Could you check a few things on this model? Use its own coordinates, in mm. Face numbers are marked on the shaded views. Give positions to 0.01 mm unless a question says otherwise; leave off trailing zeros. Order: outer loops, then holes, each group sorted by start corner. A loop starts at its lowest first (then second) coordinate and runs counter-clockwise, first axis right, second up. Notation, with made-up numbers: (-38.5, -13) - (-12.5, -13) arc R12 cw to (-12.5, 3) - close; hole circle Ø9 at (87, 76.25). An arc over 180 degrees is marked (long way). One line per question, with ' | ' between items. Start each with the question number.
1. Imagine slicing it at A-A (z = 0). Please give me the cut outline in (x, y).
2. Imagine slicing it at D-D (z = 3.25). Please give me the cut outline in (x, y), and give its area (3 significant figures).
3. I need wall thicknesses on probe 1 along Z at (x, y) = (2.4, 0); probe 2 along Y at (x, z) = (1.75, 1.75); probe 3 along Z at (x, y) = (0.45, 3.5). Which ranges of each line are inside material? Lowest first, please. Write a range as from..to.
4. For P1, Ø0.9, axis at y = 0, z = 0, coming from the +X side; P2, Ø1.5, axis at x = 1, z = -2.5, coming from the -Y side, each with a flat end and sliding along its axis, tell me the tip position at first contact or that it passes through.
5. If we mould it in two halves opening along Z, with no side actions, what happens to the marked faces 1, 2, 3 and 4? For each: released by +Z, released by -Z, zero draft, split by the parting line, or undercut.
```python
from build123d import *

# Parameters (mm, degrees)
SKETCH1_R                 = 5
SKETCH1_R_2               = 1.5
BOSS_EXTRUDE1_DEPTH       = 3
SKETCH2_W                 = 0.580440463
SKETCH2_H                 = 2
SKETCH2_W_2               = 2
SKETCH2_H_2               = 0.580440463
BOSS_EXTRUDE2_DEPTH       = 3
CHAMFER3_SIZE             = 0.2
CHAMFER4_SIZE             = 0.2
BOSS_EXTRUDE3_OUTLINE_R   = 1.5
BOSS_EXTRUDE3_OUTLINE_R_2 = 0.75
BOSS_EXTRUDE3_DEPTH       = 3


# Read off the part's stored shape, not the designer's step: Boss-Extrude3
with BuildPart() as part:
    # Sketch1 → Boss-Extrude1 (new body)
    with BuildSketch(Plane(origin=(0, 0, 0), x_dir=(0, 0, -1), z_dir=(1, 0, 0))):
        Circle(SKETCH1_R)
        Circle(SKETCH1_R_2, mode=Mode.SUBTRACT)
    extrude(amount=BOSS_EXTRUDE1_DEPTH)

    # Sketch2 → Boss-Extrude2 (add)
    with BuildSketch(Plane(origin=(3, 0, 0), x_dir=(0, 0, -1), z_dir=(1, 0, 0))):
        with Locations((4.709779769, 0)):
            Rectangle(SKETCH2_W, SKETCH2_H)
        Polygon((4.242640687, -2.828427125), (2.828427125, -4.242640687), (2.417993737, -3.8322073), (3.8322073, -2.417993737), align=None)
        with Locations((0, -4.709779769)):
            Rectangle(SKETCH2_W_2, SKETCH2_H_2)
        Polygon((-2.828427125, -4.242640687), (-4.242640687, -2.828427125), (-3.8322073, -2.417993737), (-2.417993737, -3.8322073), align=None)
        with Locations((-4.709779769, 0)):
            Rectangle(SKETCH2_W, SKETCH2_H)
        Polygon((-4.242640687, 2.828427125), (-2.828427125, 4.242640687), (-2.417993737, 3.8322073), (-3.8322073, 2.417993737), align=None)
        with Locations((0, 4.709779769)):
            Rectangle(SKETCH2_W_2, SKETCH2_H_2)
        Polygon((2.828427125, 4.242640687), (4.242640687, 2.828427125), (3.8322073, 2.417993737), (2.417993737, 3.8322073), align=None)
    extrude(amount=-BOSS_EXTRUDE2_DEPTH)

    # Chamfer3
    chamfer3_edges = [part.edges().sort_by_distance(p)[0] for p in [
        (3, 0, 5),
        (3, 1, 4.949489743),
        (3, -1, 4.949489743),
        (3, 1.913417162, 4.619397663),
        (3, 2.792710979, 4.206924542),
        (3, 3.535533906, 3.535533906),
        (3, 4.206924542, 2.792710979),
        (3, 4.619397663, 1.913417162),
        (3, 4.949489743, 1),
        (3, 5, 0),
        (3, 4.949489743, -1),
        (3, 4.619397663, -1.913417162),
        (3, 1, -4.949489743),
        (3, 0, -5),
        (3, 4.206924542, -2.792710979),
        (3, 3.535533906, -3.535533906),
        (3, 2.792710979, -4.206924542),
        (3, -1, -4.949489743),
        (3, -1.913417162, -4.619397663),
        (3, -2.792710979, -4.206924542),
        (3, -3.535533906, -3.535533906),
        (3, -4.206924542, -2.792710979),
        (3, 0, 1.5),
        (3, -4.619397663, -1.913417162),
        (3, -4.949489743, -1),
        (3, -5, 0),
        (3, -4.949489743, 1),
        (3, -4.619397663, 1.913417162),
        (3, -4.206924542, 2.792710979),
        (3, -3.535533906, 3.535533906),
        (3, -2.792710979, 4.206924542),
        (3, 1.913417162, -4.619397663),
        (3, -1.913417162, 4.619397663),
    ]]
    chamfer(chamfer3_edges, length=CHAMFER3_SIZE)

    # Chamfer4
    chamfer4_edges = [part.edges().sort_by_distance(p)[0] for p in [
        (0, -1, 4.949489743),
        (0, 0, 5),
        (0, 1, 4.949489743),
        (0, 1.913417162, -4.619397663),
        (0, 1.913417162, 4.619397663),
        (0, 2.792710979, 4.206924542),
        (0, 3.535533906, 3.535533906),
        (0, 4.206924542, 2.792710979),
        (0, 4.619397663, 1.913417162),
        (0, 1, -4.949489743),
        (0, 4.949489743, 1),
        (0, 5, 0),
        (0, 4.949489743, -1),
        (0, 0, -5),
        (0, -1, -4.949489743),
        (0, 4.619397663, -1.913417162),
        (0, 4.206924542, -2.792710979),
        (0, 3.535533906, -3.535533906),
        (0, 2.792710979, -4.206924542),
        (0, -1.913417162, -4.619397663),
        (0, -2.792710979, -4.206924542),
        (0, -3.535533906, -3.535533906),
        (0, -4.206924542, -2.792710979),
        (0, 0, 1.5),
        (0, -4.619397663, -1.913417162),
        (0, -4.949489743, -1),
        (0, -5, 0),
        (0, -4.949489743, 1),
        (0, -4.619397663, 1.913417162),
        (0, -4.206924542, 2.792710979),
        (0, -3.535533906, 3.535533906),
        (0, -2.792710979, 4.206924542),
        (0, -1.913417162, 4.619397663),
    ]]
    chamfer(chamfer4_edges, length=CHAMFER4_SIZE)

    # Boss-Extrude3 outline → Boss-Extrude3 (add)
    with BuildSketch(Plane.YZ):
        Circle(BOSS_EXTRUDE3_OUTLINE_R)
        Circle(BOSS_EXTRUDE3_OUTLINE_R_2, mode=Mode.SUBTRACT)
    extrude(amount=BOSS_EXTRUDE3_DEPTH)


solid = part.part
```
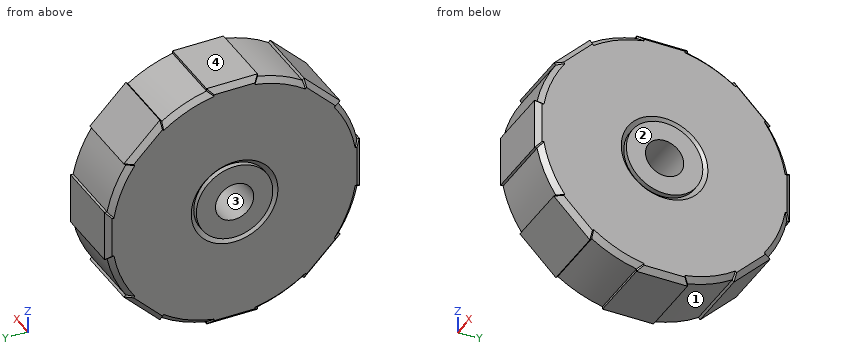
Results found:
1) outline: (0, -4.8) - (0.2, -5) - (2.8, -5) - (3, -4.8) - (3, -1.7) - (2.8, -1.5) - (3, -1.5) - (3, -0.75) - (0, -0.75) - (0, -1.5) - (0.2, -1.5) - (0, -1.7) - close; (0, 0.75) - (3, 0.75) - (3, 1.5) - (2.8, 1.5) - (3, 1.7) - (3, 4.8) - (2.8, 5) - (0.2, 5) - (0, 4.8) - (0, 1.7) - (0.2, 1.5) - (0, 1.5) - close
2) outline: (0, -3.54) - (0.2, -3.82) - (2.8, -3.82) - (3, -3.54) - (3, 3.54) - (2.8, 3.82) - (0.2, 3.82) - (0, 3.54) - close | area: 22.8 mm2
3) probe 1: z = -5..-0.75, 0.75..5 | probe 2: y = -4.68..4.68 | probe 3: z = -3.57..3.57
4) P1: passes through | P2: stops at y = -4.68
5) face 1: released by -Z | face 2: zero draft | face 3: undercut | face 4: released by +Z
